Could you check a few things on this model? Use its own coordinates, in mm. A direction names the side the tool comes from. Round coordinates to 2 decimals unless told otherwise and drop trailing zeros. Order: outer loops, then holes, each group sorted by start corner. A loop starts at its lowest first (then second) coordinate and runs counter-clockwise, first axis right, second up. Notation, with made-up numbers: (15.5, 34) - (19.5, 34) arc R21 ccw to (19.5, 49) - close; hole circle Ø11 at (17.5, 25). An arc over 180 degrees is marked (long way). Return JSON: item names as keys, results as strings. Group by question number.
from build123d import *

# Parameters (mm, degrees)
SKETCH2_W           = 80
SKETCH2_H           = 80
BOSS_EXTRUDE1_DEPTH = 5
SKETCH9_R           = 3
BOSS_EXTRUDE3_DEPTH = 5
SKETCH10_R          = 1.75
CUT_EXTRUDE6_DEPTH  = 58.445626465
SKETCH11_R          = 2.9
BOSS_EXTRUDE4_DEPTH = 80
SKETCH12_W          = 80
SKETCH12_H          = 80
SKETCH12_W_2        = 7
SKETCH12_H_2        = 20
CUT_EXTRUDE7_DEPTH  = 64.118935352


with BuildPart() as part:
    # Sketch2 → Boss-Extrude1 (new body)
    with BuildSketch(Plane(origin=(0, 0, 0), x_dir=(1, 0, 0), z_dir=(0, 1, 0))):
        Rectangle(SKETCH2_W, SKETCH2_H)
    extrude(amount=BOSS_EXTRUDE1_DEPTH)

    # Sketch9 → Boss-Extrude3 (add)
    with BuildSketch(Plane.XZ):
        with Locations(Location((-34.5, 34.5, 0), (0, 0, 270))):
            Circle(SKETCH9_R)
        with Locations(Location((34.5, 34.5, 0), (0, 0, 270))):
            Circle(SKETCH9_R)
        with Locations(Location((-34.5, -34.5, 0), (0, 0, 270))):
            Circle(SKETCH9_R)
        with Locations(Location((34.5, -34.5, 0), (0, 0, 270))):
            Circle(SKETCH9_R)
    extrude(amount=BOSS_EXTRUDE3_DEPTH)

    # Sketch10 → Cut-Extrude6 (cut, through all)
    with BuildSketch(Plane.XZ.offset(5)):
        with Locations(Location((-34.5, -34.5, 0), (0, 0, 270))):
            Circle(SKETCH10_R)
        with Locations(Location((-34.5, 34.5, 0), (0, 0, 270))):
            Circle(SKETCH10_R)
        with Locations(Location((34.5, 34.5, 0), (0, 0, 270))):
            Circle(SKETCH10_R)
        with Locations(Location((34.5, -34.5, 0), (0, 0, 270))):
            Circle(SKETCH10_R)
    extrude(amount=-CUT_EXTRUDE6_DEPTH, mode=Mode.SUBTRACT)

    # Sketch11 → Boss-Extrude4 (add)
    with BuildSketch(Plane(origin=(40, 0, 0), x_dir=(0, 0, -1), z_dir=(1, 0, 0))):
        with BuildLine():
            Line((-10, 5), (-10, 23))
            ThreePointArc((-10, 23), (0, 33), (10, 23))
            Line((10, 23), (10, 5))
            Line((10, 5), (-10, 5))
        make_face()
        with Locations((0, 23)):
            Circle(SKETCH11_R, mode=Mode.SUBTRACT)
    extrude(amount=-BOSS_EXTRUDE4_DEPTH)

    # Sketch12 → Cut-Extrude7 (cut, through all)
    with BuildSketch(Plane(origin=(0, 5, 0), x_dir=(1, 0, 0), z_dir=(0, 1, 0))):
        Rectangle(SKETCH12_W, SKETCH12_H)
        Rectangle(SKETCH12_W_2, SKETCH12_H_2, mode=Mode.SUBTRACT)
    extrude(amount=CUT_EXTRUDE7_DEPTH, mode=Mode.SUBTRACT)


solid = part.part
1) If I drill on line 1 along X through (y, z) = (-1.75, -34.5); line 2 along Z through (x, y) = (34, -2); line 3 along X through (y, z) = (27, 2), over which ranges is the centre line in solid material (lowest first)? Write a range as from..to.
2) I want a section at C-C, the plane z = 0. List the corners of the cut face in (x, y) for me, plus the area to 3 significant figures.
3) We'd pull the mould along X, two halves only. Please class faces 1 (the cylindrical face through (34.6, -2.5, -31.5)), 2 (the flat face through (40, 2, 1)), 3 (the cylindrical face through (0.05, 20.17, 0.63)), 4 (the cylindrical face through (-34.4, -2.5, -31.5)): +X half, -X half, draft (parallel to the pull), parting line (faces both ways), or undercut.
4) For faces 5 (the flat face through (0, 14, 10)), 6 (the cylindrical face through (-34.42, -0.07, -32.75)), 7 (the flat face through (3.5, 19, 0)), 8 (the flat face through (-1, 0, -1)), 9 (the cylindrical face through (0, 33, 0)), which set-ups out of +Z, -Z, +X, -X, +Y, -Y let a thin tool reach every point of the face, with its end or its side?
5) I want a section at B-B, the plane x = -34.5. List the corners of the cut face in (y, z) for me, plus the area to 3 significant figures.
6) I want a section at D-D, the plane y = 22. List the corners of the cut face in (x, z) for me, plus the area to 3 significant figures.
7) Will these pins go through, and if not, where does the flat tip stop? pin 1 (6 mm diameter, centred on x = -26, y = -0.5, fed in from -Z); pin 2 (10 mm diameter, centred on x = 0.5, z = -15, fed in from -Y); pin 3 (10 mm diameter, centred on x = 24.5, z = 15, fed in from +Y); pin 4 (6.5 mm diameter, centred on y = 23, z = 0, fed in from -X).
8) I want a section at A-A, the plane z = -34.5. List the corners of the cut face in (x, y) for me, plus the area to 3 significant figures.
Outcome:
{
 "1": {"line 1": "-37.5..-36.25, -32.75..-31.5, 31.5..32.75, 36.25..37.5", "line 2": "-37.46..-36.18, -32.82..-31.54, 31.54..32.82, 36.18..37.46", "line 3": "-3.5..3.5"},
 "2": {"outline": "(-40, 0) - (40, 0) - (40, 5) - (3.5, 5) - (3.5, 20.1) - (-3.5, 20.1) - (-3.5, 5) - (-40, 5) - close; (-3.5, 25.9) - (3.5, 25.9) - (3.5, 33) - (-3.5, 33) - close", "area": "555 mm^2"},
 "3": {"face 1": "undercut", "face 2": "+X half", "face 3": "draft", "face 4": "undercut"},
 "4": {"face 5": "+Z, +X, -X, +Y", "face 6": "+Y, -Y", "face 7": "+Z, -Z, +X, +Y", "face 8": "-Y", "face 9": "+X, -X, +Y"},
 "5": {"outline": "(-5, -37.5) - (0, -37.5) - (0, -40) - (5, -40) - (5, -36.25) - (-5, -36.25) - close; (-5, -32.75) - (5, -32.75) - (5, 32.75) - (-5, 32.75) - (-5, 31.5) - (0, 31.5) - (0, -31.5) - (-5, -31.5) - close; (-5, 36.25) - (5, 36.25) - (5, 40) - (0, 40) - (0, 37.5) - (-5, 37.5) - close", "area": "390 mm^2"},
 "6": {"outline": "(-3.5, -10) - (3.5, -10) - (3.5, -2.72) - (-3.5, -2.72) - close; (-3.5, 2.72) - (3.5, 2.72) - (3.5, 10) - (-3.5, 10) - close", "area": "102 mm^2"},
 "7": {"pin 1": "z = -40", "pin 2": "y = 0", "pin 3": "y = 5", "pin 4": "x = -3.5"},
 "8": {"outline": "(-40, 0) - (-37.5, 0) - (-37.5, -5) - (-36.25, -5) - (-36.25, 5) - (-40, 5) - close; (-32.75, -5) - (-31.5, -5) - (-31.5, 0) - (31.5, 0) - (31.5, -5) - (32.75, -5) - (32.75, 5) - (-32.75, 5) - close; (36.25, -5) - (37.5, -5) - (37.5, 0) - (40, 0) - (40, 5) - (36.25, 5) - close", "area": "390 mm^2"}
}
